Verification items for this drawing (mm, ordinates from the low corner). Give positions to 0.01 mm unless a question says otherwise; leave off trailing zeros. Order: outer loops, then holes, each group sorted by start corner. A loop starts at its lowest first (then second) coordinate and runs counter-clockwise, first axis right, second up.
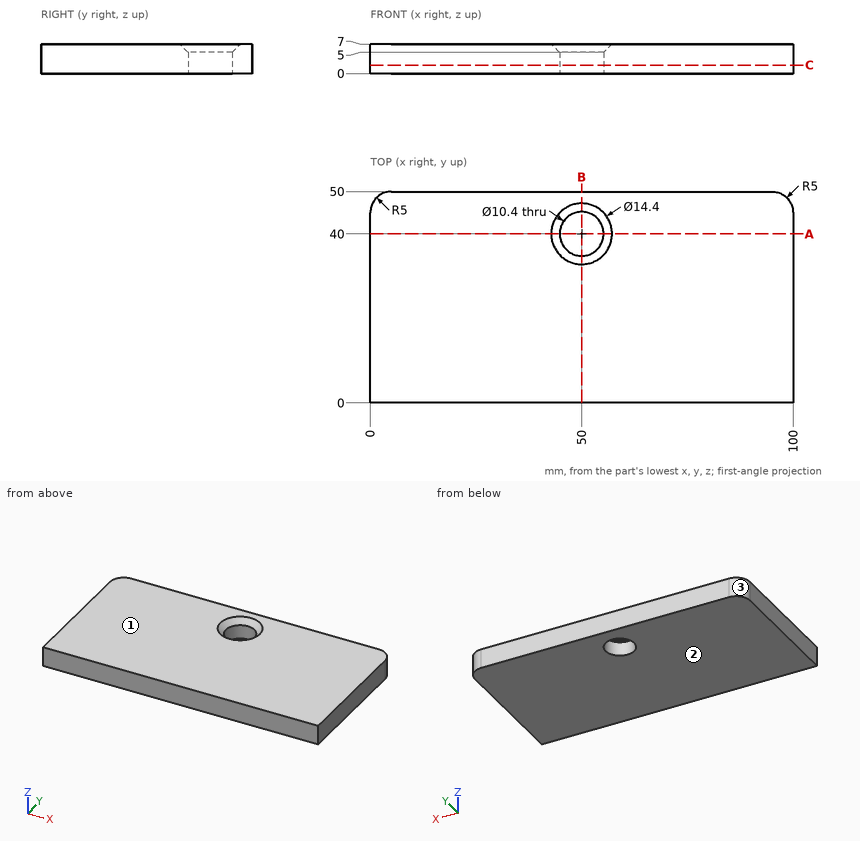
Q1. Thickness scan on L1, parallel to Y at x = 50, z = 1.7; L2, parallel to X at y = 44, z = 3.5; L3, parallel to Y at x = 51.5, z = 6.25. Record the ranges inside material, lowest first.
Q2. Cross-section at B-B, the plane x = 50. Record the boundary of the cut face in (y, z), and give its area (3 significant figures).
Q3. Cross-section at C-C, the plane z = 2. Record the boundary of the cut face in (x, y).
Q4. Release check for a two-part mould opening along Z. For the marked faces 1, 2 and 3 record: pulls with the +Z half, pulls with the -Z half, needs draft (parallel to the pull), parting line crosses it, or undercut.
Q5. Cross-section at A-A, the plane y = 40. Record the boundary of the cut face in (x, z), and give its area (3 significant figures).
Answers follow:
1. L1: y = 0 to 34.8, 45.2 to 50
1. L2: x = 0 to 46.68, 53.32 to 100
1. L3: y = 0 to 33.73, 46.27 to 50
2. outline: (0, 0) - (34.8, 0) - (34.8, 5) - (32.8, 7) - (0, 7) - close; (45.2, 0) - (50, 0) - (50, 7) - (47.2, 7) - (45.2, 5) - close
2. area: 273 mm2
3. outline: (0, 0) - (100, 0) - (100, 45) arc R5 ccw to (95, 50) - (5, 50) arc R5 ccw to (0, 45) - close; hole circle Ø10.4 at (50, 40)
4. face 1: pulls with the +Z half
4. face 2: pulls with the -Z half
4. face 3: needs draft
5. outline: (0, 0) - (44.8, 0) - (44.8, 5) - (42.8, 7) - (0, 7) - close; (55.2, 0) - (100, 0) - (100, 7) - (57.2, 7) - (55.2, 5) - close
5. area: 623 mm2
